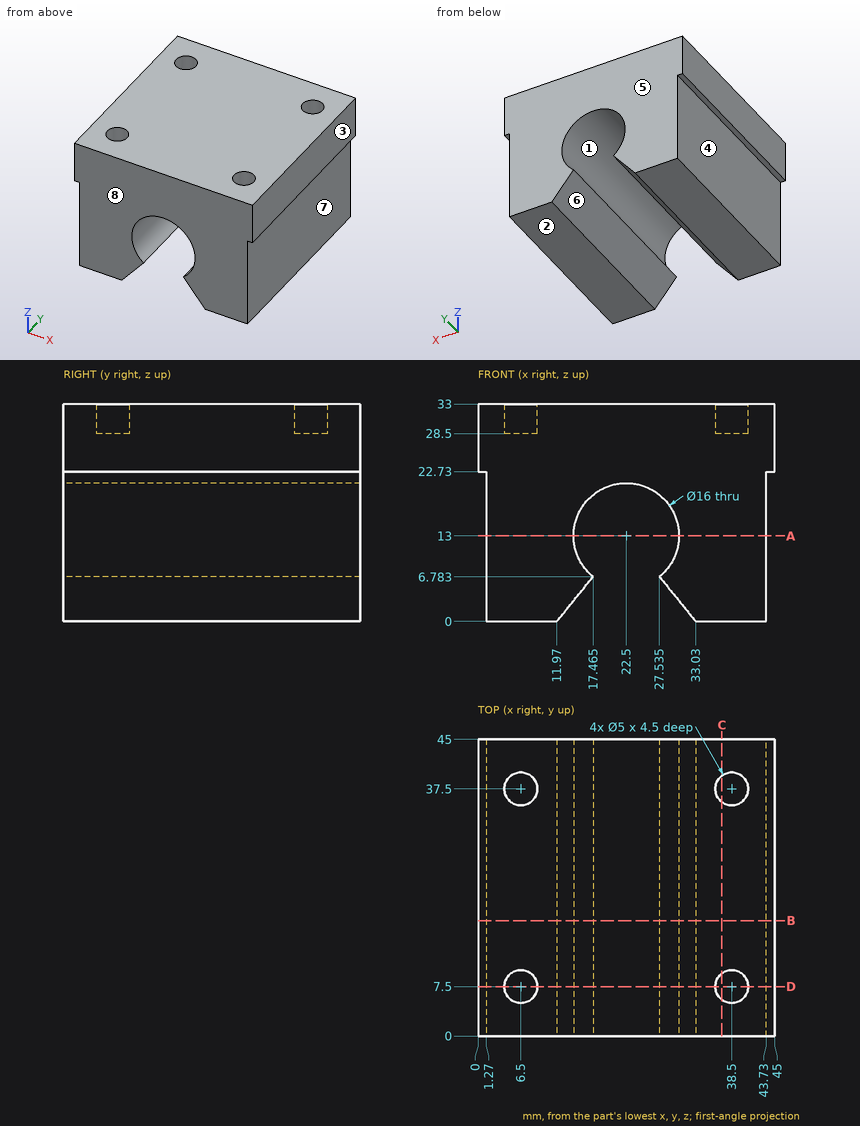
Part print with two shaded views. Sizes in mm from the minimum x, y, z corner. A direction names the side the tool comes from. Round coordinates to 2 decimals unless told otherwise and drop trailing zeros. Loops run counter-clockwise (first coordinate to the right, second up) from the corner with the lowest first, then second, coordinate; pieces in that order, holes last. Notation, with made-up numbers: (-0.5, 86) - (12.5, 86) arc R10 ccw to (12.5, 99) - close; hole circle Ø3 at (69, 11). An arc over 180 degrees is marked (long way). Put each result on its own line as item: value.
1. Slice it at D-D on y = 7.5. List the corners of the cut face in (x, z) (1 decimal), and give its area (3 significant figures).
Geometry check:
outline: (0, 22.7) - (1.3, 22.7) - (1.3, 0) - (12, 0) - (17.5, 6.8) arc R8 cw (long way) to (27.5, 6.8) - (33, 0) - (43.7, 0) - (43.7, 22.7) - (45, 22.7) - (45, 33) - (41, 33) - (41, 28.5) - (36, 28.5) - (36, 33) - (9, 33) - (9, 28.5) - (4, 28.5) - (4, 33) - (0, 33) - close
area: 1,090 mm²
2. Slice it at C-C on x = 37. List the corners of the cut face in (y, z).
Geometry check:
outline: (0, 0) - (45, 0) - (45, 33) - (39.5, 33) - (39.5, 28.5) - (35.5, 28.5) - (35.5, 33) - (9.5, 33) - (9.5, 28.5) - (5.5, 28.5) - (5.5, 33) - (0, 33) - close
3. Two-plate mould, pull along X, no slides. Class the marked faces 1, 2 and 3: released by +X, released by -X, zero draft, split by the parting line, or undercut.
Geometry check:
face 1: undercut
face 2: zero draft
face 3: released by +X
4. 3-axis set-ups, long thin cutter, end or side, ignore diameter. For the marked faces 4, 5, 6, 7 and 8: which of +Z, -Z, +X, -X, +Y, -Y reach the whole face in a straight line?
Geometry check:
face 4: -Z, -X, +Y, -Y
face 5: +Z, -Z, +X, -X, +Y
face 6: -Z, +Y, -Y
face 7: -Z, +X, +Y, -Y
face 8: +Z, -Z, +X, -X, -Y
5. Slice it at A-A on z = 13. List the corners of the cut face in (x, y).
Geometry check:
outline: (1.27, 0) - (14.5, 0) - (14.5, 45) - (1.27, 45) - close; (30.5, 0) - (43.73, 0) - (43.73, 45) - (30.5, 45) - close
6. Wall check: line 1 (Y direction, x = 38.5, z = 31.15); line 2 (X direction, y = 29.5, z = 13); line 3 (X direction, y = 37, z = 31). Give the ranges that are in metal, low to high.
Geometry check:
line 1: 0 to 5, 10 to 35, 40 to 45
line 2: 1.27 to 14.5, 30.5 to 43.73
line 3: 0 to 4.05, 8.95 to 36.05, 40.95 to 45
7. Slice it at B-B on y = 17.5. List the corners of the cut face in (x, z) (1 decimal).
Geometry check:
outline: (0, 22.7) - (1.3, 22.7) - (1.3, 0) - (12, 0) - (17.5, 6.8) arc R8 cw (long way) to (27.5, 6.8) - (33, 0) - (43.7, 0) - (43.7, 22.7) - (45, 22.7) - (45, 33) - (0, 33) - close
8. Pin check, flat tips, straight feed: P1, Ø1.4, axis at x = 0.5, y = 30.5, coming from the -Z side; P2, Ø6.5, axis at x = 38.5, y = 7.5, coming from the +Z side; P3, Ø1.5, axis at x = 37.5, y = 38, coming from the +Z side; P4, Ø14.5, axis at x = 22.5, z = 13, coming from the +Y side. Stop position of each tip, or through.
Geometry check:
P1: z = 22.73
P2: z = 33
P3: z = 28.5
P4: through
